```python
from build123d import *

# Parameters (mm, degrees)
SKETCH1_R           = 1.55
BOSS_EXTRUDE1_DEPTH = 1.55
FILLET1_R           = 2.75
FILLET2_R           = 4
SKETCH2_W           = 4.295601851
SKETCH2_H           = 3.758651621
SKETCH2_W_2         = 10.067816841
SKETCH2_H_2         = 9.880137001
SKETCH2_W_3         = 1.533271648
SKETCH2_H_3         = 2.732965052
SKETCH2_W_4         = 4.933230252
SKETCH2_H_4         = 3.296205995
BOSS_EXTRUDE2_DEPTH = 1.3
SKETCH3_W           = 2.751869936
SKETCH3_H           = 1.431170206
BOSS_EXTRUDE3_DEPTH = 1
SKETCH5_W           = 15.136693504
SKETCH5_H           = 14.663476204
SKETCH5_W_2         = 3.786204625
SKETCH5_H_2         = 3.249978942
SKETCH5_W_3         = 1.854200636
SKETCH5_H_3         = 2.974253985
SKETCH5_W_4         = 1.124105555
SKETCH5_H_4         = 1.832284905
SKETCH5_W_5         = 2.879214045
SKETCH5_H_5         = 1.227517325
SKETCH5_W_6         = 1.439607023
SKETCH5_H_6         = 2.644088496
SKETCH5_W_7         = 1.062909192
SKETCH5_H_7         = 1.901844146
BOSS_EXTRUDE5_DEPTH = 1.36
SKETCH6_W           = 1.377049396
SKETCH6_H           = 0.847415013
SKETCH6_H_2         = 0.715006417
SKETCH6_H_3         = 0.741488137
LED_DEPTH           = 0.4


with BuildPart() as part:
    # Sketch1 → Boss-Extrude1 (new body)
    with BuildSketch(Plane(origin=(0, 0, 0), x_dir=(1, 0, 0), z_dir=(0, 1, 0))):
        Polygon((-12.5, 18), (-18, 18), (-18, -18), (-12.5, -18), (-12.5, -13.78), (12.5, -13.78), (12.5, -18), (18, -18), (18, 18), (12.5, 18), (12.5, 13.78), (-12.5, 13.78), align=None)
        with Locations(Location((-15.25, -15.25, 0), (0, 0, 90))):
            Circle(SKETCH1_R, mode=Mode.SUBTRACT)
        with Locations(Location((15.25, -15.25, 0), (0, 0, 90))):
            Circle(SKETCH1_R, mode=Mode.SUBTRACT)
        with Locations(Location((-15.25, 15.25, 0), (0, 0, 90))):
            Circle(SKETCH1_R, mode=Mode.SUBTRACT)
        with Locations(Location((15.25, 15.25, 0), (0, 0, 90))):
            Circle(SKETCH1_R, mode=Mode.SUBTRACT)
    extrude(amount=BOSS_EXTRUDE1_DEPTH)

    # Fillet1
    fillet1_edges = [part.edges().sort_by_distance(p)[0] for p in [
        (-12.5, 0.775, -18),
        (-18, 0.775, -18),
        (-18, 0.775, 18),
        (-12.5, 0.775, 18),
        (12.5, 0.775, 18),
        (18, 0.775, 18),
        (18, 0.775, -18),
        (12.5, 0.775, -18),
    ]]
    fillet(fillet1_edges, radius=FILLET1_R - 0.0001)  # a hair under: the kernel refuses the full size

    # Fillet2
    fillet2_edges = [part.edges().sort_by_distance(p)[0] for p in [
        (12.5, 0.775, -13.78),
        (-12.5, 0.775, -13.78),
        (12.5, 0.775, 13.78),
        (-12.5, 0.775, 13.78),
    ]]
    fillet(fillet2_edges, radius=FILLET2_R)

    # Sketch2 → Boss-Extrude2 (add)
    with BuildSketch(Plane(origin=(0, 1.55, 0), x_dir=(1, 0, 0), z_dir=(0, 1, 0))):
        with Locations((-12.61578846, -4.950009947)):
            Rectangle(SKETCH2_W, SKETCH2_H)
        with Locations((0.64017038, -0.742248111)):
            Rectangle(SKETCH2_W_2, SKETCH2_H_2)
        with Locations((12.011098572, 4.06360308)):
            Rectangle(SKETCH2_W_3, SKETCH2_H_3)
        with Locations((-13.471552891, 7.404508181)):
            Rectangle(SKETCH2_W_4, SKETCH2_H_4)
    extrude(amount=BOSS_EXTRUDE2_DEPTH)

    # Sketch3 → Boss-Extrude3 (add)
    with BuildSketch(Plane(origin=(0, 2.85, 0), x_dir=(1, 0, 0), z_dir=(0, 1, 0))):
        with Locations((-13.589010754, 7.578480249)):
            Rectangle(SKETCH3_W, SKETCH3_H)
    extrude(amount=BOSS_EXTRUDE3_DEPTH)

    # Sketch5 → Boss-Extrude5 (add)
    with BuildSketch(Plane.XZ):
        with Locations((-10.431653248, 0.794028878)):
            Rectangle(SKETCH5_W, SKETCH5_H)
        with Locations((12.566755317, -8.673138409)):
            Rectangle(SKETCH5_W_2, SKETCH5_H_2)
        with Locations((13.887030707, -2.780074404)):
            Rectangle(SKETCH5_W_3, SKETCH5_H_3)
        with Locations((11.235705782, -2.742909061)):
            Rectangle(SKETCH5_W_4, SKETCH5_H_4)
        with Locations((-1.024391328, -3.653442734)):
            Rectangle(SKETCH5_W_5, SKETCH5_H_5)
        with Locations((-0.304587816, 2.835875505)):
            Rectangle(SKETCH5_W_6, SKETCH5_H_6)
        with Locations((16.130877107, -8.512116058)):
            Rectangle(SKETCH5_W_7, SKETCH5_H_7)
    extrude(amount=BOSS_EXTRUDE5_DEPTH)

    # Sketch6 → LED (add)
    with BuildSketch(Plane(origin=(0, 1.55, 0), x_dir=(1, 0, 0), z_dir=(0, 1, 0))):
        with Locations((-15.541502651, 4.54846251)):
            Rectangle(SKETCH6_W, SKETCH6_H)
        with Locations((-15.541502651, 3.317062568)):
            Rectangle(SKETCH6_W, SKETCH6_H_2)
        with Locations((-15.541502651, 1.940013173)):
            Rectangle(SKETCH6_W, SKETCH6_H_3)
    extrude(amount=LED_DEPTH)


solid = part.part
```
For this review, take the finished solid that the model builds, in its own axes (mm). A direction names the side the tool comes from. Coordinates: 2 decimals unless noted, no trailing zeros. Order: outer loops, then holes, each group sorted by start corner. A loop starts at its lowest first (then second) coordinate and runs counter-clockwise, first axis right, second up. Notation, with made-up numbers: (-25.5, 58) -> (23.5, 58) arc R25 cw to (23.5, 86) -> close; hole circle Ø5 at (-22.5, 20.5). An arc over 180 degrees is marked (long way). Answer as CSV lines item,"result".
Q1. For faces 5 (the face through (16, -1, -9.463)), 6 (the face through (-12.213, 3.3, -7.6)), 7 (the face through (-14, 3, -8.294)), 8 (the face through (0, 1, 13.78)), 9 (the face through (-1.024, -1, 3)), list the 3-axis set-ups (+Z, -Z, +X, -X, +Y, -Y) from which the entire face can be reached by the end or side of a thin tool; tool diameter is ignored.
Model answer:
face 5,"-Z, +X, -Y"
face 6,"+Z, -Z, +X, +Y"
face 7,"-Z, +X, -X, +Y"
face 8,"+Z, +Y, -Y"
face 9,"+Z, -Y"
Q2. Wall thickness on line 1 along Z through (x, y) = (-15.25, 0.5); line 2 along X through (y, z) = (0.95, -15.25); line 3 along Y through (x, z) = (-2, 11.5): over which ranges is each line inside the solid? List them lowest first. Write a range as [from, to].
Model answer:
line 1,"z = [-18, -16.8], [-13.7, 13.7], [16.8, 18]"
line 2,"x = [-18, -16.8], [-13.7, -12.09], [12.09, 13.7], [16.8, 18]"
line 3,"y = [0, 1.55]"
Q3. We need section C-C (y = 0.5). Count the separate pieces of the cut face and the enclosed holes in it, plus the area to 3 significant figures.
Model answer:
separate pieces,"1"
enclosed holes,"4"
area,"1,050 mm2"
Q4. Draft analysis for pull direction X (two halves, no side actions). For faces 1 (the face through (-14, 3.85, -8)), 2 (the face through (17.22, 0.79, 17.17)), 3 (the face through (14.46, -1, -9)), 4 (the face through (0, 1, -13.78)), state which applies: released by +X, released by -X, zero draft, split by the parting line, or undercut.
Model answer:
face 1,"zero draft"
face 2,"released by +X"
face 3,"undercut"
face 4,"undercut"
Q5. We need section B-B (z = 0.5). State the section outline as (x, y) points.
Model answer:
outline,"(-18, -1.36) -> (-2.86, -1.36) -> (-2.86, 0) -> (18, 0) -> (18, 1.55) -> (5.67, 1.55) -> (5.67, 2.85) -> (-4.39, 2.85) -> (-4.39, 1.55) -> (-18, 1.55) -> close"
Q6. Clearance check with flat-ended pins moving along their axes: pin 1 Ø4 at (x, z) = (-1.5, -9.5) entering from -Y; pin 2 Ø10 at (x, z) = (-14.5, 6.5) entering from +Y; pin 3 Ø1.5 at (x, z) = (-2.5, -13.5) entering from +Y; pin 4 Ø3 at (x, z) = (-15.25, 15.25) entering from +Y. State where each tip first meets the part, or that it passes through.
Model answer:
pin 1,"stops at y = 0"
pin 2,"stops at y = 2.85"
pin 3,"stops at y = 1.55"
pin 4,"passes through"
Q7. We need section D-D (z = -12.5). State the section outline as (x, y) points, plus the area to 3 significant figures.
Model answer:
outline,"(-18, 0) -> (18, 0) -> (18, 1.55) -> (-18, 1.55) -> close"
area,"55.8 mm2"
Q8. We need section A-A (x = -6.5). State the section outline as (y, z) points.
Model answer:
outline,"(-1.36, -6.54) -> (0, -6.54) -> (0, -13.78) -> (1.55, -13.78) -> (1.55, 13.78) -> (0, 13.78) -> (0, 8.13) -> (-1.36, 8.13) -> close"
